Input: part model. Units: mm. Frame: model coordinates. A direction names the side the tool comes from. Coordinates: 2 decimals unless noted, no trailing zeros. Order: outer loops, then holes, each group sorted by start corner. A loop starts at its lowest first (then second) coordinate and runs counter-clockwise, first axis right, second up. Notation, with made-up numbers: M 44.25,33.25 L 77.25,33.25 A7 cw 77.25,42.25 Z; hole C 3.5,46 d8. An arc over 180 degrees is marked long. Answer in a Markdown table with one row per item.
from build123d import *

# Parameters (mm, degrees)
F0_W         = 100
F0_H         = 10
F1_DEPTH     = 200
F2_W         = 10
F2_H         = 70
F3_DEPTH     = 70
F5_DEPTH     = 70
F7_DEPTH     = 20
F8_T1_DEPTH  = 200
F8_T3_DEPTH  = 93
F8_T5_DEPTH  = 93
F8_S9_W      = 2
F8_S9_H      = 2
F8_T10_DEPTH = 2
F8_S15_W     = 2
F8_S15_H     = 2
F8_T16_DEPTH = 2
F8_T22_DEPTH = 73
F8_T27_DEPTH = 73
F8_T32_DEPTH = 73
F8_T37_DEPTH = 73


# Not quite as in the source:
# - a fillet or chamfer that OpenCascade refuses, or shapes differently, is made with other operations: its cross-section is extruded or revolved along the edge and cut away or added


with BuildPart() as f1:
    # F0 (on Right) → F1 (new body)
    with BuildSketch(Plane.YZ):
        Polygon((5, -100), (5, 100), (-5, 100), (-5, 23.2), (-5, 13.2), (-5, -100), align=None)
        with Locations((-55, 18.2)):
            Rectangle(F0_W, F0_H)
    extrude(amount=F1_DEPTH)

    # F2 (on face) → F3 (join)
    with BuildSketch(Plane.XZ.offset(5)):
        with Locations((100, -21.8)):
            Rectangle(F2_W, F2_H)
    extrude(amount=F3_DEPTH)

    # F4 (on face) → F5 (cut)
    with BuildSketch(Plane(origin=(95, 0, 0), x_dir=(0, -1, 0), z_dir=(-1, 0, 0))):
        Polygon((75, -56.8), (75, 13.2), (5, -56.8), align=None)
    extrude(amount=-F5_DEPTH, mode=Mode.SUBTRACT)

    # F6 (on face) → F7 (cut)
    with BuildSketch(Plane.XZ.offset(5)):
        with BuildLine():
            Line((15, 80.75), (15, 85))
            Line((15, 85), (19.25, 85))
            ThreePointArc((19.25, 85), (11.99479618, 88.00520382), (15, 80.75))
        make_face()
        with BuildLine():
            Line((19.25, 85), (15, 85))
            Line((15, 85), (15, 80.75))
            ThreePointArc((15, 80.75), (18.00520382, 81.99479618), (19.25, 85))
        make_face()
        with BuildLine():
            ThreePointArc((189.25, 85), (185, 89.25), (180.75, 85))
            Line((180.75, 85), (185, 85))
            Line((185, 85), (185, 80.75))
            ThreePointArc((185, 80.75), (188.00520382, 81.99479618), (189.25, 85))
        make_face()
        with BuildLine():
            Line((185, 85), (180.75, 85))
            ThreePointArc((180.75, 85), (181.99479618, 81.99479618), (185, 80.75))
            Line((185, 80.75), (185, 85))
        make_face()
        with BuildLine():
            ThreePointArc((189.25, -85), (188.00520382, -81.99479618), (185, -80.75))
            Line((185, -80.75), (185, -85))
            Line((185, -85), (180.75, -85))
            ThreePointArc((180.75, -85), (185, -89.25), (189.25, -85))
        make_face()
        with BuildLine():
            Line((185, -85), (185, -80.75))
            ThreePointArc((185, -80.75), (181.99479618, -81.99479618), (180.75, -85))
            Line((180.75, -85), (185, -85))
        make_face()
        with BuildLine():
            Line((15, -85), (15, -80.75))
            ThreePointArc((15, -80.75), (11.99479618, -88.00520382), (19.25, -85))
            Line((19.25, -85), (15, -85))
        make_face()
        with BuildLine():
            ThreePointArc((19.25, -85), (18.00520382, -81.99479618), (15, -80.75))
            Line((15, -80.75), (15, -85))
            Line((15, -85), (19.25, -85))
        make_face()
    extrude(amount=-F7_DEPTH, mode=Mode.SUBTRACT)

    # F8: fillet of radius 2 on 7 edges, made by hand

    # F8_s2 → F8_t1 (join)
    with BuildSketch(Plane.YZ):
        with BuildLine():
            ThreePointArc((-5, 25.2), (-5.5857864376, 23.7857864376), (-7, 23.2))
            Line((-7, 23.2), (-5, 23.2))
            Line((-5, 23.2), (-5, 25.2))
        make_face()
    extrude(amount=F8_T1_DEPTH)

    # F8_s4 → F8_t3 (join)
    with BuildSketch(Plane.YZ):
        with BuildLine():
            ThreePointArc((-5, 11.2), (-5.5857864376, 12.6142135624), (-7, 13.2))
            Line((-7, 13.2), (-5, 13.2))
            Line((-5, 13.2), (-5, 11.2))
        make_face()
    extrude(amount=F8_T3_DEPTH)

    # F8_s6 → F8_t5 (join)
    with BuildSketch(Plane.YZ.offset(107)):
        with BuildLine():
            ThreePointArc((-5, 11.2), (-5.5857864376, 12.6142135624), (-7, 13.2))
            Line((-7, 13.2), (-5, 13.2))
            Line((-5, 13.2), (-5, 11.2))
        make_face()
    extrude(amount=F8_T5_DEPTH)


with BuildPart() as f8_tool8:
    # F8_s9 → F8_t10 (new body)
    with BuildSketch(Plane.XZ.offset(7)):
        with Locations((94, 12.2)):
            Rectangle(F8_S9_W, F8_S9_H)
    extrude(amount=-F8_T10_DEPTH)

    # F8_s11 → F8_t12 (revolve, cut)
    with BuildSketch(Plane(origin=(93, -7, 11.2), x_dir=(-0.7071067812, 0, -0.7071067812), z_dir=(0.7071067812, 0, -0.7071067812))):
        with BuildLine():
            ThreePointArc((0, -2), (2, 0), (0, 2))
            Line((0, 2), (0, -2))
        make_face()
    revolve(axis=Axis((93, -7, 11.2), (0, 1, 0)), mode=Mode.SUBTRACT)


with BuildPart() as f1_1:
    add(f1.part)

    # F8_t7: union F8_tool8
    add(f8_tool8.part)


with BuildPart() as f8_tool14:
    # F8_s15 → F8_t16 (new body)
    with BuildSketch(Plane.YZ.offset(107)):
        with Locations((-6, 12.2)):
            Rectangle(F8_S15_W, F8_S15_H)
    extrude(amount=-F8_T16_DEPTH)

    # F8_s17 → F8_t18 (revolve, cut)
    with BuildSketch(Plane(origin=(107, -7, 11.2), x_dir=(0, -0.7071067812, -0.7071067812), z_dir=(0, 0.7071067812, -0.7071067812))):
        with BuildLine():
            ThreePointArc((0, -2), (2, 0), (0, 2))
            Line((0, 2), (0, -2))
        make_face()
    revolve(axis=Axis((107, -7, 11.2), (-1, 0, 0)), mode=Mode.SUBTRACT)


with BuildPart() as f1_2:
    add(f1_1.part)

    # F8_t13: union F8_tool14
    add(f8_tool14.part)


with BuildPart() as f8_tool20:
    # F8_s21 → F8_t22 (new body)
    with BuildSketch(Plane.XY.offset(-61.8)):
        with BuildLine():
            ThreePointArc((107, -5), (105.5857864376, -5.5857864376), (105, -7))
            Line((105, -7), (105, -5))
            Line((105, -5), (107, -5))
        make_face()
    extrude(amount=F8_T22_DEPTH)

    split(bisect_by=Plane(origin=(0, -30.9, -30.9), x_dir=(1, 0, 0), z_dir=(0, 0.7071067812, 0.7071067812)), keep=Keep.TOP)


with BuildPart() as f1_3:
    add(f1_2.part)

    # F8_t19: union F8_tool20
    add(f8_tool20.part)


with BuildPart() as f8_tool25:
    # F8_s26 → F8_t27 (new body)
    with BuildSketch(Plane.XY.offset(11.2)):
        with BuildLine():
            ThreePointArc((93, -5), (94.4142135624, -5.5857864376), (95, -7))
            Line((95, -7), (95, -5))
            Line((95, -5), (93, -5))
        make_face()
    extrude(amount=-F8_T27_DEPTH)

    split(bisect_by=Plane(origin=(0, -30.9, -30.9), x_dir=(1, 0, 0), z_dir=(0, 0.7071067812, 0.7071067812)), keep=Keep.TOP)


with BuildPart() as f1_4:
    add(f1_3.part)

    # F8_t24: union F8_tool25
    add(f8_tool25.part)


with BuildPart() as f8_tool30:
    # F8_s31 → F8_t32 (new body)
    with BuildSketch(Plane.XZ.offset(7)):
        with BuildLine():
            ThreePointArc((93, 13.2), (94.4142135624, 12.6142135624), (95, 11.2))
            Line((95, 11.2), (95, 13.2))
            Line((95, 13.2), (93, 13.2))
        make_face()
    extrude(amount=F8_T32_DEPTH)

    split(bisect_by=Plane(origin=(0, -30.9, -30.9), x_dir=(1, 0, 0), z_dir=(0, 0.7071067812, 0.7071067812)), keep=Keep.TOP)


with BuildPart() as f1_5:
    add(f1_4.part)

    # F8_t29: union F8_tool30
    add(f8_tool30.part)


with BuildPart() as f8_tool35:
    # F8_s36 → F8_t37 (new body)
    with BuildSketch(Plane.XZ.offset(7)):
        with BuildLine():
            ThreePointArc((107, 13.2), (105.5857864376, 12.6142135624), (105, 11.2))
            Line((105, 11.2), (105, 13.2))
            Line((105, 13.2), (107, 13.2))
        make_face()
    extrude(amount=F8_T37_DEPTH)

    split(bisect_by=Plane(origin=(0, -30.9, -30.9), x_dir=(1, 0, 0), z_dir=(0, 0.7071067812, 0.7071067812)), keep=Keep.TOP)


with BuildPart() as f1_6:
    add(f1_5.part)

    # F8_t34: union F8_tool35
    add(f8_tool35.part)


solid = f1_6.part
1) Cut plane A-A, the plane z = -13.5. Output: boundary loops of the cut face in (x, y), and give its area (3 significant figures).
Resolved:
| item | result |
|---|---|
| outline | M 0,-5 L 93,-5 A2 cw 95,-7 L 95,-48.3 L 105,-48.3 L 105,-7 A2 cw 107,-5 L 200,-5 L 200,5 L 0,5 Z |
| area | 2,430 mm2 |
2) Material intervals for probe 1 along X at (y, z) = (-1.75, -85); probe 2 along Z at (x, y) = (15, 2.5); probe 3 along Z at (x, y) = (50, -28.5), sorted ascending.
Resolved:
| item | result |
|---|---|
| probe 1 | x = 0 to 10.75, 19.25 to 180.75, 189.25 to 200 |
| probe 2 | z = -100 to -89.25, -80.75 to 80.75, 89.25 to 100 |
| probe 3 | z = 13.2 to 23.2 |
3) Cut plane B-B, the plane y = -38. Output: boundary loops of the cut face in (x, z).
Resolved:
| item | result |
|---|---|
| outline | M 0,13.2 L 93,13.2 A2 cw 95,11.2 L 95,-23.8 L 105,-23.8 L 105,11.2 A2 cw 107,13.2 L 200,13.2 L 200,23.2 L 0,23.2 Z |
4) Cut plane C-C, the plane z = 67.5. Output: boundary loops of the cut face in (x, y), and give its area (3 significant figures).
Resolved:
| item | result |
|---|---|
| outline | M 0,-5 L 200,-5 L 200,5 L 0,5 Z |
| area | 2,000 mm2 |
5) Reachability of faces 1 (the face through (105, -25, -8)), 2 (the face through (99, -5, 63)), 3 (the face through (76, -5, -44)) from +Z, -Z, +X, -X, +Y, -Y: full face, straight path, thin tool, end or side. Return the list, or none.
Resolved:
| item | result |
|---|---|
| face 1 | -Z, +X, -Y |
| face 2 | +Z, +X, -X, -Y |
| face 3 | -Z, -Y |
6) Contact query for flat-ended pins moving along their axis: pin 1 (10 mm diameter, centred on x = 61.5, y = -76, fed in from -Z); pin 2 (5 mm diameter, centred on x = 104.5, z = 45.5, fed in from -Y); pin 3 (3 mm diameter, centred on x = 46, y = -18.5, fed in from +Z). Output: stop coordinate, or through.
Resolved:
| item | result |
|---|---|
| pin 1 | stops at z = 13.2 |
| pin 2 | stops at y = -5 |
| pin 3 | stops at z = 23.2 |
